from build123d import *

# Parameters (mm, degrees)
F0_W     = 300
F0_H     = 60
F1_DEPTH = 10
F2_W     = 300
F2_H     = 10
F3_DEPTH = 300
F4_R     = 117.5
F5_DEPTH = 60.001
F6_W     = 60
F6_H     = 10
F7_DEPTH = 200


with BuildPart() as f1:
    # F0 (on Front) → F1 (new body)
    with BuildSketch(Plane.XZ):
        Rectangle(F0_W, F0_H)
        Polygon((-150, 30), (150, 30), (30, 80), (0, 80), (-30, 80), align=None)
    extrude(amount=F1_DEPTH)

    # F2 (on face) → F3 (join)
    with BuildSketch(Plane.XZ.offset(10)):
        with Locations((0, 25)):
            Rectangle(F2_W, F2_H)
    extrude(amount=F3_DEPTH)

    # F4 (on face) → F5 (cut, through all)
    with BuildSketch(Plane(origin=(0, 0, 20), x_dir=(1, 0, 0), z_dir=(0, 0, -1))):
        with Locations((0, 160)):
            Circle(F4_R)
    extrude(amount=-F5_DEPTH, mode=Mode.SUBTRACT)

    # F6 (on face) → F7 (join)
    with BuildSketch(Plane.XZ.offset(10)):
        with Locations((0, 75)):
            Rectangle(F6_W, F6_H)
    extrude(amount=F7_DEPTH)


solid = f1.part
Check sheet for the modelled part. Datum: model origin and axes. Units: mm. A direction names the side the tool comes from. Round coordinates to 2 decimals unless told otherwise and drop trailing zeros. Order: outer loops, then holes, each group sorted by start corner. A loop starts at its lowest first (then second) coordinate and runs counter-clockwise, first axis right, second up.
(1) Cross-section at D-D, the plane x = -82.5. Enter the section's corners in (y, z) (3 decimals), and give its area (3 significant figures).
(2) Access from +Z, -Z, +X, -X, +Y, -Y to the whole of each face (thin tool, end or side, straight path). Record for faces 5 (the flat face through (-2, -10, -5)), 6 (the flat face through (0, -109, 70)), 7 (the flat face through (-30, -109, 75)), 8 (the flat face through (30, -109, 75)).
(3) Cross-section at A-A, the plane x = 0. Enter the section's corners in (y, z), and give its area (3 significant figures).
(4) Cross-section at C-C, the plane y = -244. Enter the section's corners in (x, z), and give its area (3 significant figures).
(5) Go/stop test with flat-tipped pins: P1, Ø18, axis at x = -10.5, y = -97.5, coming from the -Z side; P2, Ø1, axis at x = -53, z = 36.5, coming from the +Y side; P3, Ø5, axis at y = -138.5, z = 73, coming from the -X side; P4, Ø5, axis at y = -109, z = 74, coming from the +X side. Record where each tip stops, or that it passes through.
(6) Scan lines: probe 1 along Y at (x, z) = (0, 27); probe 2 along X at (y, z) = (-160, 23); probe 3 along Y at (x, z) = (-28.5, 7). Record each from-to range of solid material in increasing order.
(7) Cross-section at B-B, the plane y = -160. Enter the section's corners in (x, z).
(8) Draft check along Z on faces 1 (the flat face through (-2, -10, 50)), 2 (the flat face through (90.84, -4.93, 54.65)), 3 (the flat face through (-2, -5, -30)), 4 (the cylindrical face through (63.167, -259.076, 24.93)). Enter one of: pulls with the +Z half, pulls with the -Z half, needs draft (parallel to the pull), parting line crosses it, or undercut.
Check sheet entries:
1. outline: (-310, 20) - (-243.666, 20) - (-243.666, 30) - (-310, 30) - close; (-76.334, 20) - (-10, 20) - (-10, -30) - (0, -30) - (0, 58.125) - (-10, 58.125) - (-10, 30) - (-76.334, 30) - close
1. area: 2,210 mm2
2. face 5: -Z, +X, -X, -Y
2. face 6: +X, -X, -Y
2. face 7: +Z, -X, -Y
2. face 8: +Z, +X, -Y
3. outline: (-310, 20) - (-277.5, 20) - (-277.5, 30) - (-310, 30) - close; (-210, 70) - (-10, 70) - (-10, 30) - (-42.5, 30) - (-42.5, 20) - (-10, 20) - (-10, -30) - (0, -30) - (0, 80) - (-210, 80) - close
3. area: 3,750 mm2
4. outline: (-150, 20) - (-82.16, 20) - (-82.16, 30) - (-150, 30) - close; (82.16, 20) - (150, 20) - (150, 30) - (82.16, 30) - close
4. area: 1,360 mm2
5. P1: stops at z = 70
5. P2: stops at y = 0
5. P3: stops at x = -30
5. P4: stops at x = 30
6. probe 1: y = -310 to -277.5, -42.5 to 0
6. probe 2: x = -150 to -117.5, 117.5 to 150
6. probe 3: y = -10 to 0
7. outline: (-150, 20) - (-117.5, 20) - (-117.5, 30) - (-150, 30) - close; (-30, 70) - (30, 70) - (30, 80) - (-30, 80) - close; (117.5, 20) - (150, 20) - (150, 30) - (117.5, 30) - close
8. face 1: undercut
8. face 2: pulls with the +Z half
8. face 3: pulls with the -Z half
8. face 4: needs draft
